Here's how the part is built. I have some questions about the finished solid (model axes, mm). A direction names the side the tool comes from. Coordinates: 2 decimals unless noted, no trailing zeros. Loops run counter-clockwise (first coordinate to the right, second up) from the corner with the lowest first, then second, coordinate; pieces in that order, holes last. Notation, with made-up numbers: (84.25, -23.5) -> (110.25, -23.5) arc R24 cw to (110.25, 4.5) -> close; hole circle Ø1 at (6.5, -39). An arc over 180 degrees is marked (long way). Answer as a JSON object with one key per item and string values. Group by question number.
Q1. I'm going to push flat-ended pins straight in: pin 1 (3 mm diameter, centred on x = -3.5, y = -3, fed in from -Z); pin 2 (4 mm diameter, centred on x = 3, z = 6.5, fed in from +Y). Where does each tip first touch, or does it pass through?
Q2. I want a section at A-A on x = 0. Write out the boundary of the cut face in (y, z), then the cut area to 3 significant figures.
Q3. On a 3-axis mill with a long thin cutter (end or side, diameter ignored), from which of +Z, -Z, +X, -X, +Y, -Y can I reach the whole of each face in a straight line? I mean faces 1 (the cylindrical face through (-0.965, -4.344, 9.874)), 2 (the cylindrical face through (-0.108, -0.488, 22.721)). Say none if no direction works.
Q4. I want a section at D-D on z = 21.75. Write out the boundary of the cut face in (x, y), then the cut area to 3 significant figures.
Q5. I want a section at C-C on z = 9. Write out the boundary of the cut face in (x, y), then the cut area to 3 significant figures.
Q6. I need wall thicknesses on line 1 (Z direction, x = -1.25, y = -1.75); line 2 (Y direction, x = 3.25, z = 18); line 3 (X direction, y = 4, z = 12.75). Which ranges of each line are inside material? Lowest first, please.
```python
from build123d import *

# Parameters (mm, degrees)
F0_R     = 4.45
F1_DEPTH = 20
F2_R     = 1
F3_R     = 0.5
F4_DEPTH = 5.519319


with BuildPart() as f1:
    # F0 (on Top) → F1 (new body)
    with BuildSketch(Plane.XY):
        Circle(F0_R)
    extrude(amount=F1_DEPTH)

    # F2
    f2_edges = [f1.edges().sort_by_distance(p)[0] for p in [
        (-4.45, 0, 20),
        (-4.45, 0, 0),
    ]]
    fillet(f2_edges, radius=F2_R)

    # F3 (on face) → F4 (join)
    with BuildSketch(Plane.XY.offset(20)):
        Circle(F3_R)
    extrude(amount=F4_DEPTH)


solid = f1.part
```
Result set:
{
 "1": {"pin 1": "stops at z = 0", "pin 2": "stops at y = 4.34"},
 "2": {"outline": "(-4.45, 1) arc R1 ccw to (-3.45, 0) -> (3.45, 0) arc R1 ccw to (4.45, 1) -> (4.45, 19) arc R1 ccw to (3.45, 20) -> (0.5, 20) -> (0.5, 25.52) -> (-0.5, 25.52) -> (-0.5, 20) -> (-3.45, 20) arc R1 ccw to (-4.45, 19) -> close", "area": "183 mm²"},
 "3": {"face 1": "+Z, -Z", "face 2": "+Z"},
 "4": {"outline": "circle Ø1 at (0, 0)", "area": "0.785 mm²"},
 "5": {"outline": "circle Ø8.9 at (0, 0)", "area": "62.2 mm²"},
 "6": {"line 1": "z = 0 to 20", "line 2": "y = -3.04 to 3.04", "line 3": "x = -1.95 to 1.95"}
}
